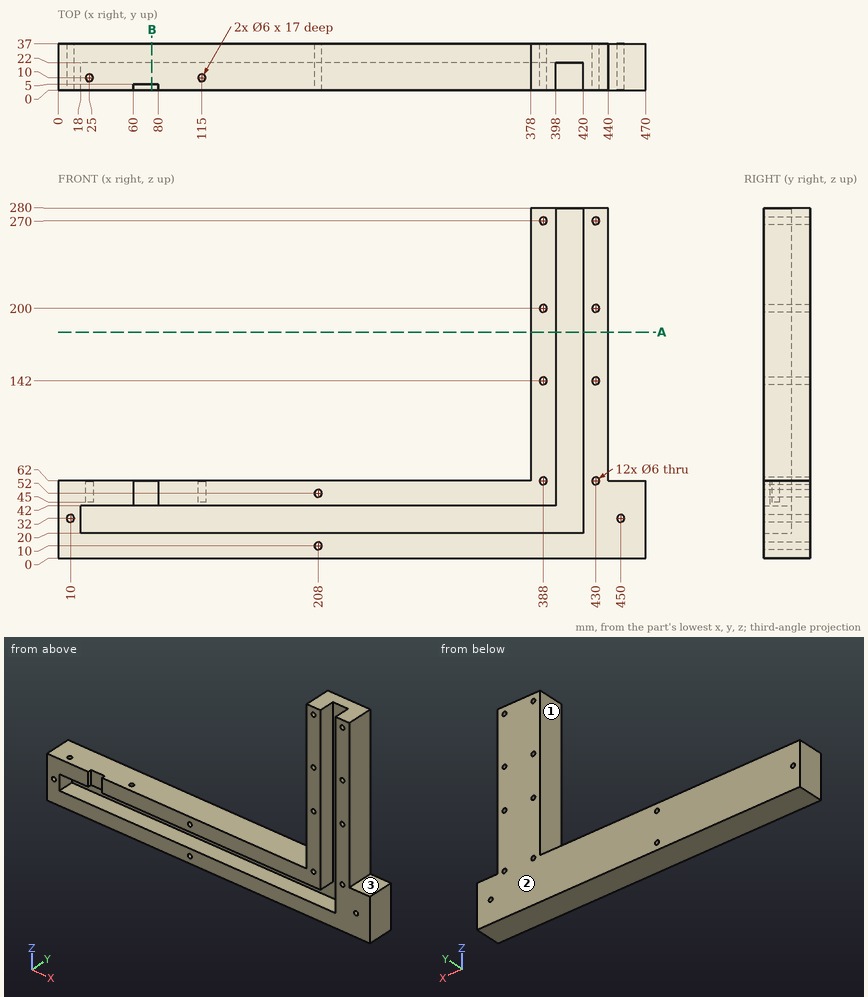
Drawing for the job (mm, zero at the part's lowest x, y, z). A direction names the side the tool comes from. Give positions to 0.01 mm unless a question says otherwise; leave off trailing zeros. Order: outer loops, then holes, each group sorted by start corner. A loop starts at its lowest first (then second) coordinate and runs counter-clockwise, first axis right, second up. Notation, with made-up numbers: M 28.25,-16 L 66.25,-16 A21 cw 66.25,21 Z; hole C 75.5,74 d6. An arc over 180 degrees is marked long. Put each result on its own line as item: value.
Item 1: Flat gauge pins, fed straight in: pin 1 Ø8 at (x, y) = (108, 5) entering from +Z; pin 2 Ø6.5 at (y, z) = (11.5, 197.5) entering from +X; pin 3 Ø18.5 at (y, z) = (9.5, 220) entering from -X. Where does each tip first touch, or does it go through?
From the geometry:
pin 1: stops at z = 62
pin 2: stops at x = 440
pin 3: stops at x = 378
Item 2: Slice it at B-B, the plane x = 75. Write the cut outline in (y, z), plus the area to 3 significant figures.
From the geometry:
outline: M 0,0 L 37,0 L 37,62 L 5,62 L 5,42 L 22,42 L 22,20 L 0,20 Z
area: 1,710 mm2
Item 3: 3-axis set-ups, long thin cutter, end or side, ignore diameter. For the marked faces 1, 2 and 3: which of +Z, -Z, +X, -X, +Y, -Y reach the whole face in a straight line?
From the geometry:
face 1: +Z, -X, +Y, -Y
face 2: +Z, -Z, +X, -X, +Y
face 3: +Z, +X, +Y, -Y
Item 4: Probe line 1 (Z direction, x = 430, y = 24); line 2 (X direction, y = 15, z = 270); line 3 (X direction, y = 13, z = 32). List the from-to ranges inside material, lowest first. Write a range as [from, to].
From the geometry:
line 1: z = [0, 59], [65, 139], [145, 197], [203, 267], [273, 280]
line 2: x = [378, 385], [391, 398], [420, 427], [433, 440]
line 3: x = [0, 7], [13, 18], [420, 447], [453, 470]
Item 5: Slice it at A-A, the plane z = 181. Write the cut outline in (x, y), plus the area to 3 significant figures.
From the geometry:
outline: M 378,0 L 398,0 L 398,22 L 420,22 L 420,0 L 440,0 L 440,37 L 378,37 Z
area: 1,810 mm2
